```python
from build123d import *

# Parameters (mm, degrees)
IZIM1_R                     = 1.5
Y_KSEKLIK_EKSTR_ZYON1_DEPTH = 1
IZIM2_R                     = 1.25
Y_KSEKLIK_EKSTR_ZYON2_DEPTH = 70
IZIM5_R                     = 1.5
IZIM5_R_2                   = 0.5
Y_KSEKLIK_EKSTR_ZYON5_DEPTH = 1.5


with BuildPart() as part:
    # Çizim1 → Yükseklik-Ekstrüzyon1 (new body, symmetric)
    with BuildSketch(Plane.XY):
        Circle(IZIM1_R)
    extrude(amount=Y_KSEKLIK_EKSTR_ZYON1_DEPTH, both=True)

    # Çizim2 → Yükseklik-Ekstrüzyon2 (add)
    with BuildSketch(Plane(origin=(0, 0, -1), x_dir=(-1, 0, 0), z_dir=(0, 0, -1))):
        Circle(IZIM2_R)
    extrude(amount=Y_KSEKLIK_EKSTR_ZYON2_DEPTH)

    # Çizim5 → Yükseklik-Ekstrüzyon5 (add, symmetric)
    with BuildSketch(Plane(origin=(0, 0, 0), x_dir=(0, 0, -1), z_dir=(1, 0, 0))):
        with Locations((72, 0)):
            Circle(IZIM5_R)
        with Locations((72, 0)):
            Circle(IZIM5_R_2, mode=Mode.SUBTRACT)
    extrude(amount=Y_KSEKLIK_EKSTR_ZYON5_DEPTH, both=True)


solid = part.part
```
Could you check a few things on this model? Use its own coordinates, in mm. A direction names the side the tool comes from. Round coordinates to 2 decimals unless told otherwise and drop trailing zeros. Loops run counter-clockwise (first coordinate to the right, second up) from the corner with the lowest first, then second, coordinate; pieces in that order, holes last. Notation, with made-up numbers: (45.25, -39) - (90.25, -39) arc R15 cw to (90.25, -24) - close; hole circle Ø4 at (10, 68.5). An arc over 180 degrees is marked (long way). Use CSV: the item, a comma, the result in double quotes.
Item 1: If we section it at B-B on x = 0: List the corners of the cut face in (y, z) for me, then the cut area to 3 significant figures.
Here are the results:
outline,"(-1.5, -1) - (-1.25, -1) - (-1.25, -71) - (-1.12, -71) arc R1.5 ccw (long way) to (1.12, -71) - (1.25, -71) - (1.25, -1) - (1.5, -1) - (1.5, 1) - (-1.5, 1) - close; hole circle Ø1 at (0, -72)"
area,"187 mm²"
Item 2: If we section it at A-A on y = 0: List the corners of the cut face in (x, z) for me, then the cut area to 3 significant figures.
Here are the results:
outline,"(-1.5, -73.5) - (1.5, -73.5) - (1.5, -72.5) - (-1.5, -72.5) - close; (-1.5, -71.5) - (1.5, -71.5) - (1.5, -70.5) - (1.25, -70.5) - (1.25, -1) - (1.5, -1) - (1.5, 1) - (-1.5, 1) - (-1.5, -1) - (-1.25, -1) - (-1.25, -70.5) - (-1.5, -70.5) - close"
area,"186 mm²"
Item 3: For faces 4 (the cylindrical face through (0.27, -1.22, -35.51)), 5 (the flat face through (1.5, -1, -72)), 6 (the cylindrical face through (-1.5, 0.07, 0.01)), which set-ups out of +Z, -Z, +X, -X, +Y, -Y let a thin tool reach every point of the face, with its end or its side?
Here are the results:
face 4,"none"
face 5,"+Z, -Z, +X, +Y, -Y"
face 6,"+Z"
Item 4: I need wall thicknesses on L1, parallel to Y at x = 0.05, z = -72; L2, parallel to X at y = 0.1, z = -62; L3, parallel to X at y = -0.75, z = -50.5. Which ranges of each line are inside material? Lowest first, please. Write a range as [from, to].
Here are the results:
L1,"y = [-1.5, -0.5], [0.5, 1.5]"
L2,"x = [-1.25, 1.25]"
L3,"x = [-1, 1]"
Item 5: If we section it at C-C on z = -14: List the corners of the cut face in (x, y) for me.
Here are the results:
outline,"circle Ø2.5 at (0, 0)"
Item 6: If we mould it in two halves opening along Z, with no side actions, what happens to faces 1 (the flat face through (0, 0, 1)), 2 (the cylindrical face through (0.02, 0.45, -73.43)), 3 (the flat face through (-1.5, -1, -72))? For each: pulls with the +Z half, pulls with the -Z half, needs draft (parallel to the pull), parting line crosses it, or undercut.
Here are the results:
face 1,"pulls with the +Z half"
face 2,"undercut"
face 3,"needs draft"
Item 7: Will these pins go through, and if not, where does the flat tip stop? pin 1 (1.5 mm diameter, centred on x = -1, y = 1, fed in from -Z); pin 2 (1.5 mm diameter, centred on y = 1, z = -46, fed in from +X).
Here are the results:
pin 1,"stops at z = -73.48"
pin 2,"stops at x = 1.22"
